Could you check a few things on this model? Use its own coordinates, in mm. Face numbers are marked on the shaded views. A direction names the side the tool comes from. Coordinates: 2 decimals unless noted, no trailing zeros. Order: outer loops, then holes, each group sorted by start corner. A loop starts at its lowest first (then second) coordinate and runs counter-clockwise, first axis right, second up. Notation, with made-up numbers: (-19, 58) -> (6, 58) arc R31 ccw to (6, 94) -> close; hole circle Ø9 at (29, 70.25). An arc over 180 degrees is marked (long way). Use a Markdown table: item, result. Add a question column.
1) If I drill on L1, parallel to X at y = 0.5, z = -1.25; L2, parallel to Y at x = -20.5, z = -1.1; L3, parallel to X at y = 0, z = -1.4, over which ranges is the centre line in solid material (lowest first)? Write a range as [from, to].
2) If we section it at D-D (y = 3.75): Write out the boundary of the cut face in (x, z).
3) If we section it at B-B (z = -1.2): Write out the boundary of the cut face in (x, y).
4) If we section it at A-A (y = 0): Write out the boundary of the cut face in (x, z).
5) Will these pins go through, and if not, where does the flat tip stop? pin 1 Ø1.6 at (x, y) = (-20.39, -0.64) entering from -Z; pin 2 Ø0.6 at (x, z) = (-18, -1.5) entering from +Y.
6) If we section it at C-C (x = -14): Write out the boundary of the cut face in (y, z).
7) Which directions (+Z, -Z, +X, -X, +Y, -Y) give clear straight access to the entire face, cutting with the end or side of a thin tool? Please do the marked faces 5, 6 and 7.
8) Thinking about a two-plate mould opening in X: for the marked faces 1, 2, 3 and 4, which applies, +X half, -X half, draft (parallel to the pull), parting line (faces both ways), or undercut?
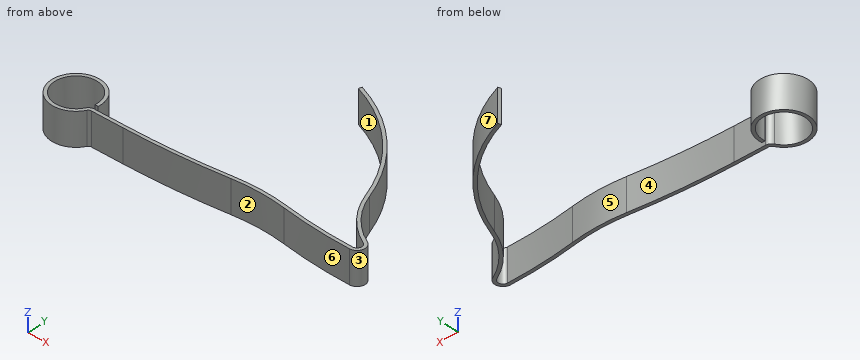
Autodesk Inventor part; units mm, degrees
ref_plane "YZ Plane" through (0, 0, 0) normal (1, 0, 0) x (0, 1, 0)
ref_plane "XZ Plane" through (0, 0, 0) normal (0, 1, 0) x (-1, 0, 0)
ref_plane "XY Plane" through (0, 0, 0) normal (0, 0, 1) x (1, 0, 0)
sketch "Sketch1" plane through (0, 0, 0) normal (0, 0, 1) x (1, 0, 0)
  arc A0 (-2.8862, -1.2447) -> (-2.6561, -0.3007) centre (-2.8862, -0.7447) ccw
  arc A1 (-7.2602, -0.8985) -> (-2.8862, -1.2447) centre (-2.8862, 26.566) ccw
  arc A2 (-5.0488, 2.4151) -> (-2.6561, -0.3007) centre (-0.3551, 4.1384) ccw
  arc A3 (-5.0488, 2.4151) -> (-11.1621, 8.4942) centre (-14.6238, -1.1004) ccw
  arc A4 (-16.9335, -1.2455) -> (-10.6071, -0.846) centre (-16.9124, 48.7131) ccw
  arc A5 (-7.2602, -0.8985) -> (-10.6071, -0.846) centre (-9.1171, -12.5575) ccw
  arc A6 (-16.9335, -1.0455) -> (-10.6324, -0.6476) centre (-16.9124, 48.7131) ccw
  arc A7 (-7.2288, -0.701) -> (-10.6324, -0.6476) centre (-9.1171, -12.5575) ccw
  arc A8 (-7.2288, -0.701) -> (-2.8862, -1.0447) centre (-2.8862, 26.566) ccw
  arc A9 (-2.8862, -1.0447) -> (-2.7481, -0.4783) centre (-2.8862, -0.7447) ccw
  arc A10 (-5.2365, 2.3461) -> (-2.7481, -0.4783) centre (-0.3551, 4.1384) ccw
  arc A11 (-5.2365, 2.3461) -> (-11.23, 8.3061) centre (-14.6238, -1.1004) ccw
  line L0 (-11.1621, 8.4942) -> (-11.23, 8.3061)
  line L1 (-5.2365, 2.3461) -> (-5.0488, 2.4151) construction
  line L2 (-2.7481, -0.4783) -> (-2.6561, -0.3007) construction
  line L3 (-5.0488, 2.4151) -> (-0.3551, 4.1384) construction
  line L4 (-0.3551, 4.1384) -> (-2.6561, -0.3007) construction
  line L5 (-11.23, 8.3061) -> (-14.6238, -1.1004) construction
  arc A12 (-18.8918, -0.7763) -> (-19.0627, -1.3505) centre (-20.3859, -0.644) ccw
  arc A13 (-18.8862, -1.2447) -> (-19.0627, -1.3505) centre (-18.8862, -1.4447) ccw
  arc A14 (-19.0927, -0.7763) -> (-19.2391, -1.2563) centre (-20.3859, -0.644) ccw
  arc A15 (-18.8861, -1.0447) -> (-19.2391, -1.2563) centre (-18.8862, -1.4447) ccw
  line L6 (-18.8862, -1.2447) -> (-16.9335, -1.2455)
  line L7 (-18.8861, -1.0447) -> (-16.9335, -1.0455)
  line L8 (-18.8862, -1.2447) -> (-2.8862, -1.2447) construction
  line L9 (-19.0927, -0.7763) -> (-18.8918, -0.7763)
  point P0 (-18.8374, -1.1048)
  dimension "d25" = 50
  dimension "d26" = 42.44
  dimension "d27" = 10
  dimension "d28" = 5
  dimension "d34" = 0.5
  dimension "d35" = 1.3
  dimension "d36" = 16
extrude "Extrusion2" add sketch "Sketch1" against normal blind 2
properties part number "scissor_spring"
Answer sheet:
| question | item | result |
|---|---|---|
| 1 | L1 | [-21.36, -21], [-19.77, -19.42], [-4.07, -3.78] |
| 1 | L2 | [-2.14, -1.94], [0.65, 0.85] |
| 1 | L3 | [-21.74, -21.52], [-19.26, -19.03], [-3.5, -3.16] |
| 2 | outline | (-5.88, -2) -> (-5.65, -2) -> (-5.65, 0) -> (-5.88, 0) -> close |
| 3 | outline | (-19.24, -1.26) arc R1.3 cw (long way) to (-19.09, -0.78) -> (-18.89, -0.78) arc R1.5 ccw (long way) to (-19.06, -1.35) arc R0.2 cw to (-18.89, -1.24) -> (-16.93, -1.25) arc R49.96 ccw to (-10.61, -0.85) arc R11.8 cw to (-7.26, -0.9) arc R27.82 ccw to (-2.89, -1.24) arc R0.5 ccw to (-2.66, -0.3) arc R5 cw to (-5.05, 2.42) arc R10.2 ccw to (-11.16, 8.49) -> (-11.23, 8.31) arc R10 cw to (-5.24, 2.35) arc R5.2 ccw to (-2.75, -0.48) arc R0.3 cw to (-2.89, -1.04) arc R27.62 cw to (-7.23, -0.7) arc R12.01 ccw to (-10.63, -0.65) arc R49.75 cw to (-16.93, -1.05) -> (-18.89, -1.04) arc R0.4 ccw to start |
| 4 | outline | (-21.74, -2) -> (-21.52, -2) -> (-21.52, 0) -> (-21.74, 0) -> close; (-19.26, -2) -> (-19.03, -2) -> (-19.03, 0) -> (-19.26, 0) -> close; (-3.5, -2) -> (-3.16, -2) -> (-3.16, 0) -> (-3.5, 0) -> close |
| 5 | pin 1 | through |
| 5 | pin 2 | y = -1.04 |
| 6 | outline | (-1.16, -2) -> (-0.96, -2) -> (-0.96, 0) -> (-1.16, 0) -> close |
| 7 | face 5 | +Z, -Z |
| 7 | face 6 | +Z, -Z, -Y |
| 7 | face 7 | +Z, -Z, +X, +Y |
| 8 | face 1 | -X half |
| 8 | face 2 | undercut |
| 8 | face 3 | +X half |
| 8 | face 4 | undercut |
